Here's the drawing with two shaded views (mm, measured from the low corner). I have some questions. A direction names the side the tool comes from. Coordinates: 2 decimals unless noted, no trailing zeros. Write each loop counter-clockwise with the first axis right and the second up, starting at its lowest first coordinate (ties: lowest second). Pieces come first, ordered by that corner, then holes.
Item 1: We'd pull the mould along Z, two halves only. Please class the marked faces 4, 5 and 6: +Z half, -Z half, draft (parallel to the pull), parting line (faces both ways), or undercut.
Item 2: If we section it at C-C (x = 60.5): Please give me the cut outline in (y, z), then the cut area to 3 significant figures.
Item 3: I'm going to push flat-ended pins straight in: pin 1 Ø6 at (y, z) = (16, 52) entering from -X; pin 2 Ø0.6 at (y, z) = (33.5, 64) entering from -X; pin 3 Ø7.5 at (x, y) = (91.5, 60) entering from -Z. Where does each tip first touch, or does it pass through?
Item 4: For the marked faces 1, 2 and 3, which set-ups out of +Z, -Z, +X, -X, +Y, -Y let a thin tool reach every point of the face, with its end or its side?
Item 5: If we section it at B-B (z = 40.5): Please give me the cut outline in (x, y), then the cut area to 3 significant figures.
Item 6: If I drill on line 1 (Z direction, x = 92, y = 59); line 2 (Z direction, x = 32, y = 6); line 3 (X direction, y = 70, z = 38), over which ranges is the centre line in solid material (lowest first)?
Item 7: If we section it at A-A (y = 23.5): Please give me the cut outline in (x, z).
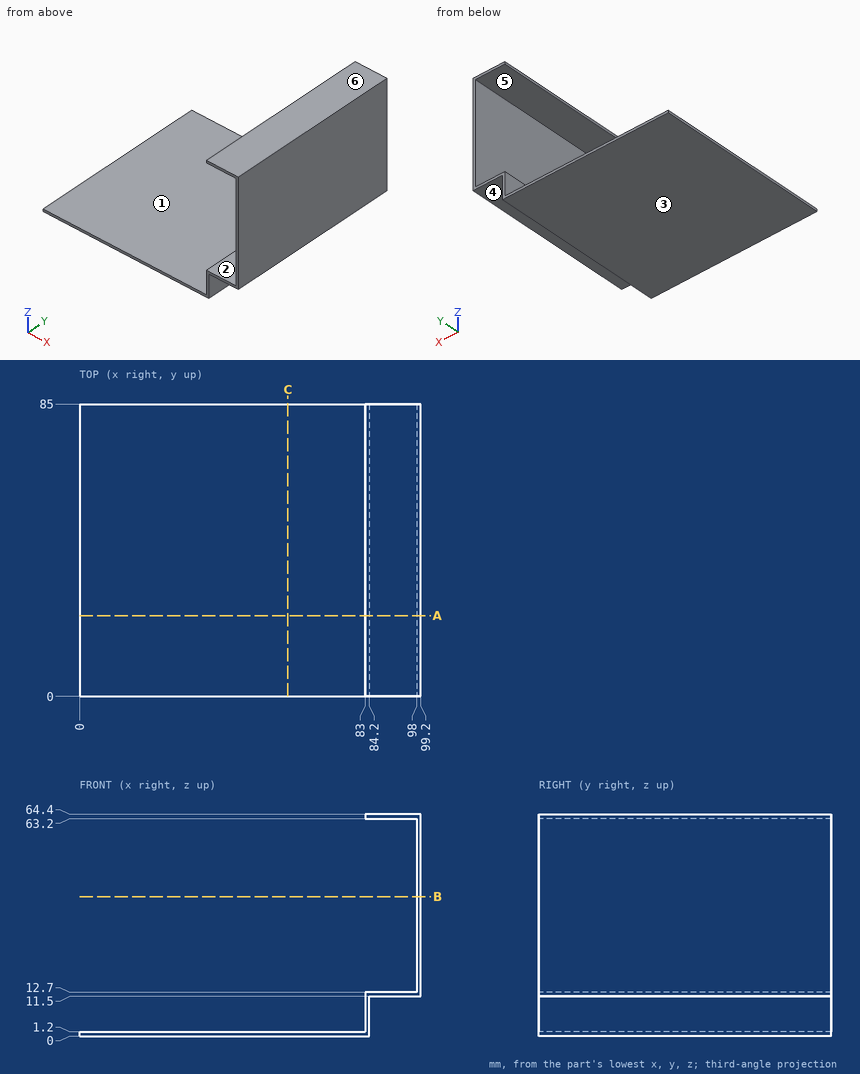
Answer list:
1. face 4: -Z half
1. face 5: undercut
1. face 6: +Z half
2. outline: (0, 0) - (85, 0) - (85, 1.2) - (0, 1.2) - close
2. area: 102 mm2
3. pin 1: stops at x = 98
3. pin 2: stops at x = 83
3. pin 3: stops at z = 11.5
4. face 1: +Z, -X, +Y, -Y
4. face 2: -X, +Y, -Y
4. face 3: -Z, +X, -X, +Y, -Y
5. outline: (98, 0) - (99.2, 0) - (99.2, 85) - (98, 85) - close
5. area: 102 mm2
6. line 1: z = 11.5 to 12.7, 63.2 to 64.4
6. line 2: z = 0 to 1.2
6. line 3: x = 98 to 99.2
7. outline: (0, 0) - (84.2, 0) - (84.2, 11.5) - (99.2, 11.5) - (99.2, 64.4) - (83, 64.4) - (83, 63.2) - (98, 63.2) - (98, 12.7) - (83, 12.7) - (83, 1.2) - (0, 1.2) - close
